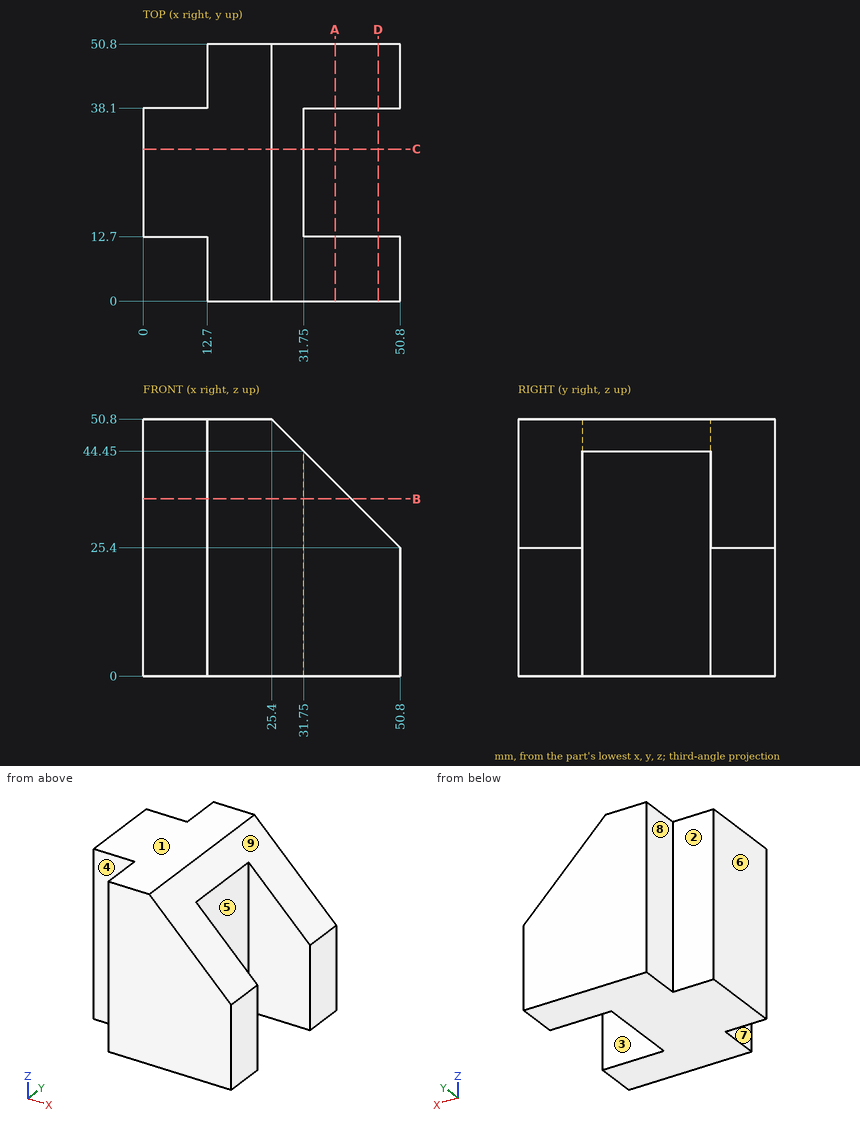
Job drawing, mm, ordinate dimensions from the low corner. One solid piece. A direction names the side the tool comes from. Round coordinates to 2 decimals unless told otherwise and drop trailing zeros. Loops run counter-clockwise (first coordinate to the right, second up) from the corner with the lowest first, then second, coordinate; pieces in that order, holes last. Notation, with made-up numbers: (2, 7.25) -> (53, 7.25) arc R36 cw to (53, 43.25) -> close; hole circle Ø9 at (81.25, 78). An arc over 180 degrees is marked (long way). Use a Markdown table: item, result.
1) Tool access for the marked faces 5, 6, 7, 8 and 9: list every direction of +Z, -Z, +X, -X, +Y, -Y with a clear straight run to the whole face (end or side of a thin tool).
The answers:
| item | result |
|---|---|
| face 5 | +Z, -Z, +X |
| face 6 | +Z, -Z, -X, +Y, -Y |
| face 7 | +Z, -Z, -X, -Y |
| face 8 | +Z, -Z, -X, +Y |
| face 9 | +Z, +X, +Y, -Y |
2) Cut at D-D, the plane x = 46.5. List the corners of the cut face in (y, z), and give its area (3 significant figures).
The answers:
| item | result |
|---|---|
| outline | (0, 0) -> (12.7, 0) -> (12.7, 29.7) -> (0, 29.7) -> close; (38.1, 0) -> (50.8, 0) -> (50.8, 29.7) -> (38.1, 29.7) -> close |
| area | 754 mm2 |
3) Probe line 1 (Y direction, x = 47.5, z = 24); line 2 (X direction, y = 30, z = 11); line 3 (Y direction, x = 12.5, z = 22.5). List the from-to ranges inside material, lowest first. Write a range as [from, to].
The answers:
| item | result |
|---|---|
| line 1 | y = [0, 12.7], [38.1, 50.8] |
| line 2 | x = [0, 31.75] |
| line 3 | y = [12.7, 38.1] |
4) Drop flat-ended pins along their axis: pin 1 Ø1 at (y, z) = (9.5, 43) entering from +X; pin 2 Ø20.5 at (y, z) = (26, 30) entering from +X; pin 3 Ø4 at (x, z) = (6.5, 23.5) entering from +Y. Give the stop position or say it passes through.
The answers:
| item | result |
|---|---|
| pin 1 | stops at x = 33.7 |
| pin 2 | stops at x = 31.75 |
| pin 3 | stops at y = 38.1 |
5) Cut at A-A, the plane x = 38. List the corners of the cut face in (y, z), and give its area (3 significant figures).
The answers:
| item | result |
|---|---|
| outline | (0, 0) -> (12.7, 0) -> (12.7, 38.2) -> (0, 38.2) -> close; (38.1, 0) -> (50.8, 0) -> (50.8, 38.2) -> (38.1, 38.2) -> close |
| area | 970 mm2 |
6) Cut at B-B, the plane z = 35. List the corners of the cut face in (x, y), and give its area (3 significant figures).
The answers:
| item | result |
|---|---|
| outline | (0, 12.7) -> (12.7, 12.7) -> (12.7, 0) -> (41.2, 0) -> (41.2, 12.7) -> (31.75, 12.7) -> (31.75, 38.1) -> (41.2, 38.1) -> (41.2, 50.8) -> (12.7, 50.8) -> (12.7, 38.1) -> (0, 38.1) -> close |
| area | 1,530 mm2 |
7) Pull direction Y, two halves, no side cores. Call the marked faces 1, 2, 3 and 4: pulls with the +Y half, pulls with the -Y half, needs draft (parallel to the pull), parting line crosses it, or undercut.
The answers:
| item | result |
|---|---|
| face 1 | needs draft |
| face 2 | pulls with the +Y half |
| face 3 | undercut |
| face 4 | pulls with the -Y half |
8) Cut at C-C, the plane y = 30. List the corners of the cut face in (x, z).
The answers:
| item | result |
|---|---|
| outline | (0, 0) -> (31.75, 0) -> (31.75, 44.45) -> (25.4, 50.8) -> (0, 50.8) -> close |
